Study the drawing (mm; zero at the part's minimum x, y, z) and answer. A direction names the side the tool comes from. Give positions to 0.01 mm unless a question says otherwise; leave off trailing zeros. Loops run counter-clockwise (first coordinate to the right, second up) from the corner with the lowest first, then second, coordinate; pieces in that order, holes last. Notation, with made-up numbers: (42.25, 1) - (53.25, 1) arc R25 cw to (53.25, 38) - close; hole circle Ø9 at (-7, -23.75). An arc over 180 degrees is marked (long way). Write item = value, one per line. Start each with the question number.
1) The part is cut by section B-B on x = 34.9. Write down the section's boundary in (y, z).
2) Flat-ended cylindrical pins translate along their axes: P1, Ø1, axis at x = 21, z = 13, coming from the +Y side; P2, Ø4, axis at y = 9.5, z = 9, coming from the -X side; P3, Ø6.5, axis at x = 3.05, z = 3.75, coming from the -Y side; P4, Ø4, axis at x = 3.05, z = 11.25, coming from the -Y side. Find the tip coordinate at first contact, or state that the pin passes through.
3) The part is cut by section C-C on z = 5. Write down the section's boundary in (x, y), plus the area to 3 significant figures.
4) The part is cut by section A-A on x = 3.05. Write down the section's boundary in (y, z), plus the area to 3 significant figures.
5) Consider probe 1 along X at (y, z) = (20.1, 3.75); probe 2 along Z at (x, y) = (3, 20); probe 3 along Y at (x, z) = (12, 5.25). Determine where each line is inside the solid, lowest interval first.
6) Which of the six approach directions +Z, -Z, +X, -X, +Y, -Y give full straight-line access (tool end or side, diameter ignored) to the marked faces 1, 2, 3, 4 and 5?
7) The part is cut by section D-D on z = 7.5. Write down the section's boundary in (x, y).
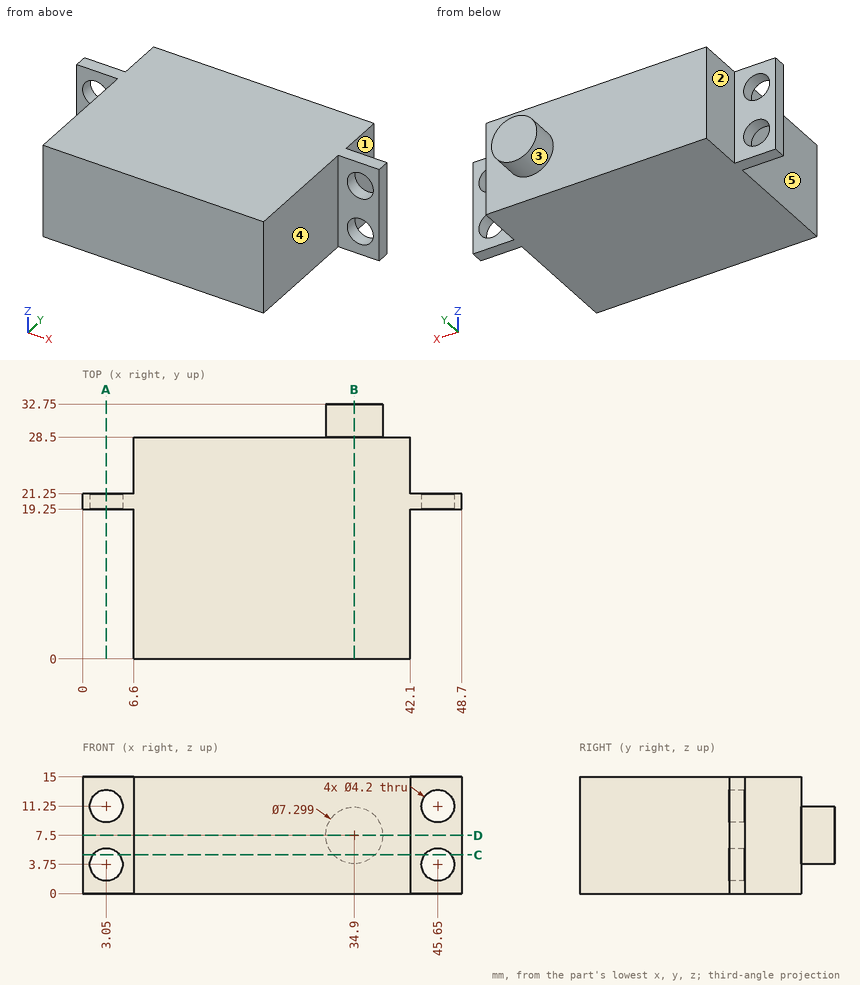
Answer below:
q1.outline = (0, 0) - (28.5, 0) - (28.5, 3.85) - (32.75, 3.85) - (32.75, 11.15) - (28.5, 11.15) - (28.5, 15) - (0, 15) - close
q2.P1 = 28.5
q2.P2 = 6.6
q2.P3 = 19.25
q2.P4 = through
q3.outline = (0, 19.25) - (1.36, 19.25) - (1.36, 21.25) - (0, 21.25) - close; (4.74, 19.25) - (6.6, 19.25) - (6.6, 0) - (42.1, 0) - (42.1, 19.25) - (43.96, 19.25) - (43.96, 21.25) - (42.1, 21.25) - (42.1, 28.5) - (37.56, 28.5) - (37.56, 32.75) - (32.24, 32.75) - (32.24, 28.5) - (6.6, 28.5) - (6.6, 21.25) - (4.74, 21.25) - close; (47.34, 19.25) - (48.7, 19.25) - (48.7, 21.25) - (47.34, 21.25) - close
q3.area = 1,050 mm2
q4.outline = (19.25, 0) - (21.25, 0) - (21.25, 1.65) - (19.25, 1.65) - close; (19.25, 5.85) - (21.25, 5.85) - (21.25, 9.15) - (19.25, 9.15) - close; (19.25, 13.35) - (21.25, 13.35) - (21.25, 15) - (19.25, 15) - close
q4.area = 13.2 mm2
q5.probe_1 = 0 to 0.95, 5.15 to 43.55, 47.75 to 48.7
q5.probe_2 = 0 to 1.65, 5.85 to 9.15, 13.35 to 15
q5.probe_3 = 0 to 28.5
q6.face_1 = +Z, -Z, +X, +Y
q6.face_2 = +Z, -Z, -X, +Y
q6.face_3 = +Y
q6.face_4 = +Z, -Z, +X, -Y
q6.face_5 = +Z, -Z, -X, -Y
q7.outline = (0, 19.25) - (6.6, 19.25) - (6.6, 0) - (42.1, 0) - (42.1, 19.25) - (48.7, 19.25) - (48.7, 21.25) - (42.1, 21.25) - (42.1, 28.5) - (38.55, 28.5) - (38.55, 32.75) - (31.25, 32.75) - (31.25, 28.5) - (6.6, 28.5) - (6.6, 21.25) - (0, 21.25) - close
